Autodesk Inventor part; units mm, degrees
ref_plane "YZ Plane" through (0, 0, 0) normal (1, 0, 0) x (0, 1, 0)
ref_plane "XZ Plane" through (0, 0, 0) normal (0, 1, 0) x (-1, 0, 0)
ref_plane "XY Plane" through (0, 0, 0) normal (0, 0, 1) x (1, 0, 0)
sketch "Sketch4" plane through (0, 0, 0) normal (0, 0, 1) x (1, 0, 0)
  line L0 (0, 0) -> (1.5, 0)
  line L1 (1.5, 0) -> (1.5, -1)
  line L2 (1.5, -1) -> (2.5, -1)
  line L3 (2.5, -1) -> (2.5, 1)
  line L4 (2.5, 1) -> (0, 1)
  line L5 (0, 1) -> (0, 0)
  dimension "d22" = 1.5
  dimension "d23" = 1
  dimension "d24" = 1
  dimension "d25" = 2
extrude "Extrusion4" add sketch "Sketch4" along normal blind 10
sketch "Sketch5" plane through (1.5, -1, 0) normal (0, -1, 0) x (1, 0, 0)
  line L0 (0, 0) -> (1, 0)
  line L1 (1, 0) -> (1, 10)
  line L2 (0, 10) -> (1, 10)
  line L3 (0, 0) -> (0, 10)
  point P0 (-1.5, 0)
extrude "Extrusion5" add sketch "Sketch5" along normal blind 3.5
sketch "Sketch6" plane through (0, 0, 0) normal (-1, 0, 0) x (0, 0, 1)
  line L0 (0, 0) -> (10, 0)
  line L1 (1.29, 0.8) -> (1.69, 0.8)
  line L2 (1.69, 0.8) -> (1.69, 0.2)
  line L3 (1.69, 0.2) -> (1.29, 0.2)
  line L4 (1.29, 0.2) -> (1.29, 0.8)
  line L5 (3.63, 0.8) -> (4.03, 0.8)
  line L6 (4.03, 0.8) -> (4.03, 0.2)
  line L7 (4.03, 0.2) -> (3.63, 0.2)
  line L8 (3.63, 0.2) -> (3.63, 0.8)
  line L9 (5.97, 0.8) -> (6.37, 0.8)
  line L10 (6.37, 0.8) -> (6.37, 0.2)
  line L11 (6.37, 0.2) -> (5.97, 0.2)
  line L12 (5.97, 0.2) -> (5.97, 0.8)
  line L13 (0, 1) -> (0, 0)
  line L14 (10, 1) -> (10, 0)
  line L15 (8.31, 0.8) -> (8.71, 0.8)
  line L16 (8.71, 0.8) -> (8.71, 0.2)
  line L17 (8.71, 0.2) -> (8.31, 0.2)
  line L18 (8.31, 0.2) -> (8.31, 0.8)
  line L19 (0, 1) -> (10, 1)
  dimension "d30" = 0.4
  dimension "d31" = 0.6
  dimension "d32" = 0.4
  dimension "d33" = 0.6
  dimension "d36" = 0.4
  dimension "d37" = 0.6
  dimension "d38" = 1.94
  dimension "d40" = 0.2
  dimension "d41" = 0.2
  dimension "d42" = 0.2
  dimension "d49" = 1.29
  dimension "d50" = 1.94
  dimension "d51" = 0.4
  dimension "d52" = 0.6
  dimension "d53" = 0.2
  dimension "d54" = 1.94
  dimension "d55" = 1.29
  dimension "d80" = 0.2
extrude "Extrusion6" add sketch "Sketch6" along normal blind 3.5 contours L1 L2 L3 L4 | L5 L6 L7 L8 | L9 L10 L11 L12 | L15 L16 L17 L18
chamfer "Chamfer5" distance 0.15 distance2 0.5 1 edges at (-3.5, 0.2, 1.49) measured on face at (-3.5, 0.6, 1.4233)
chamfer "Chamfer6" distance 0.15 distance2 0.5 1 edges at (-3.5, 0.8, 1.49) measured on face at (-3.5, 0.65, 1.4233)
chamfer "Chamfer7" distance 0.15 distance2 0.5 1 edges at (-3.5, 0.2, 3.83) measured on face at (-3.5, 0.6, 3.7633)
chamfer "Chamfer8" distance 0.15 distance2 0.5 1 edges at (-3.5, 0.8, 3.83) measured on face at (-3.5, 0.65, 3.7633)
chamfer "Chamfer9" distance 0.15 distance2 0.5 1 edges at (-3.5, 0.2, 6.17) measured on face at (-3.5, 0.6, 6.1033)
chamfer "Chamfer10" distance 0.15 distance2 0.5 1 edges at (-3.5, 0.8, 6.17) measured on face at (-3.5, 0.65, 6.1033)
chamfer "Chamfer11" distance 0.15 distance2 0.5 1 edges at (-3.5, 0.8, 8.51) measured on face at (-3.5, 0.4, 8.5767)
chamfer "Chamfer12" distance 0.15 distance2 0.5 1 edges at (-3.5, 0.2, 8.51) measured on face at (-3.5, 0.35, 8.5767)
sketch "Sketch7" plane through (1.5, -4.5, 0) normal (0, -1, 0) x (1, 0, 0)
  line L0 (0, 10) -> (0, 0)
  line L1 (0.8, 8.71) -> (0.2, 8.71)
  line L2 (0.2, 8.71) -> (0.2, 8.31)
  line L3 (0.2, 8.31) -> (0.8, 8.31)
  line L4 (0.8, 8.31) -> (0.8, 8.71)
  line L5 (0.8, 6.37) -> (0.2, 6.37)
  line L6 (0.2, 6.37) -> (0.2, 5.97)
  line L7 (0.2, 5.97) -> (0.8, 5.97)
  line L8 (0.8, 5.97) -> (0.8, 6.37)
  line L9 (0.8, 4.03) -> (0.2, 4.03)
  line L10 (0.2, 4.03) -> (0.2, 3.63)
  line L11 (0.2, 3.63) -> (0.8, 3.63)
  line L12 (0.8, 3.63) -> (0.8, 4.03)
  line L13 (0.8, 1.69) -> (0.2, 1.69)
  line L14 (0.2, 1.69) -> (0.2, 1.29)
  line L15 (0.2, 1.29) -> (0.8, 1.29)
  line L16 (0.8, 1.29) -> (0.8, 1.69)
  point P0 (-1.5, 0)
  dimension "d81" = 0.6
  dimension "d82" = 0.4
  dimension "d83" = 0.4
  dimension "d84" = 0.4
  dimension "d85" = 0.4
  dimension "d86" = 0.2
extrude "Extrusion7" cut sketch "Sketch7" against normal blind 3.7
chamfer "Chamfer13" distance 0.15 angle 45 4 edges at (2, -4.5, 4.03) (2.3, -4.5, 3.83) (2, -4.5, 3.63) (1.7, -4.5, 3.83)
chamfer "Chamfer14" distance 0.15 angle 45 4 edges at (2, -4.5, 1.69) (2.3, -4.5, 1.49) (2, -4.5, 1.29) (1.7, -4.5, 1.49)
chamfer "Chamfer15" distance 0.15 angle 45 4 edges at (2.3, -4.5, 6.17) (2, -4.5, 6.37) (1.7, -4.5, 6.17) (2, -4.5, 5.97)
chamfer "Chamfer16" distance 0.15 angle 45 4 edges at (2, -4.5, 8.31) (2.3, -4.5, 8.51) (2, -4.5, 8.71) (1.7, -4.5, 8.51)
properties part number "Pin Connector Curved"
Verification items for the finished model (mm, model axes). A direction names the side the tool comes from. Coordinates: 2 decimals unless noted, no trailing zeros. Order: outer loops, then holes, each group sorted by start corner. A loop starts at its lowest first (then second) coordinate and runs counter-clockwise, first axis right, second up.
1. Sectioned sample at A-A, the plane y = -1. Record the cut outline in (x, z), and give its area (3 significant figures).
Results found:
outline: (1.5, 0) - (2.5, 0) - (2.5, 10) - (1.5, 10) - close; hole (1.7, 1.29) - (2.3, 1.29) - (2.3, 1.69) - (1.7, 1.69) - close; hole (1.7, 3.63) - (2.3, 3.63) - (2.3, 4.03) - (1.7, 4.03) - close; hole (1.7, 5.97) - (2.3, 5.97) - (2.3, 6.37) - (1.7, 6.37) - close; hole (1.7, 8.31) - (2.3, 8.31) - (2.3, 8.71) - (1.7, 8.71) - close
area: 9.04 mm2
2. Go/stop test with flat-tipped pins: pin 1 Ø1 at (x, z) = (-1, 7.5) entering from +Y; pin 2 Ø1.5 at (y, z) = (-3.5, 3.5) entering from -X; pin 3 Ø0.7 at (x, y) = (-2, 0.5) entering from +Z. Record where each tip stops, or that it passes through.
Results found:
pin 1: passes through
pin 2: stops at x = 1.5
pin 3: stops at z = 8.71
3. Sectioned sample at B-B, the plane x = -2.15. Record the cut outline in (y, z), and give its area (3 significant figures).
Results found:
outline: (0.2, 1.29) - (0.8, 1.29) - (0.8, 1.69) - (0.2, 1.69) - close; (0.2, 3.63) - (0.8, 3.63) - (0.8, 4.03) - (0.2, 4.03) - close; (0.2, 5.97) - (0.8, 5.97) - (0.8, 6.37) - (0.2, 6.37) - close; (0.2, 8.31) - (0.8, 8.31) - (0.8, 8.71) - (0.2, 8.71) - close
area: 0.960 mm2
4. Sectioned sample at D-D, the plane x = 0.3. Record the cut outline in (y, z).
Results found:
outline: (0, 0) - (1, 0) - (1, 10) - (0, 10) - close
5. Sectioned sample at C-C, the plane z = 5. Record the cut outline in (x, y), and give its area (3 significant figures).
Results found:
outline: (0, 0) - (1.5, 0) - (1.5, -4.5) - (2.5, -4.5) - (2.5, 1) - (0, 1) - close
area: 7.00 mm2
6. Release check for a two-part mould opening along Z. For faces 1 (the face through (2, -1, 0)), 2 (the face through (0, 0.5, 4.9)), 3 (the face through (2.5, -2, 5)), 4 (the face through (2, -1, 10)) record: +Z half, -Z half, draft (parallel to the pull), parting line (faces both ways), or undercut.
Results found:
face 1: -Z half
face 2: undercut
face 3: draft
face 4: +Z half
7. Scan lines: line 1 (Z direction, x = -1.95, y = 0.6); line 2 (X direction, y = -1.35, z = 1.5); line 3 (Y direction, x = 1.2, z = 8.75). Record each from-to range of solid material in increasing order.
Results found:
line 1: z = 1.29 to 1.69, 3.63 to 4.03, 5.97 to 6.37, 8.31 to 8.71
line 2: x = 1.5 to 1.7, 2.3 to 2.5
line 3: y = 0 to 1
8. Set-up check for faces 5 (the face through (1, 0, 5)), 6 (the face through (1, 1, 5)): record each of +Z, -Z, +X, -X, +Y, -Y from which the full face is reachable in a straight line by a thin tool's end or side.
Results found:
face 5: +Z, -Z, -X, -Y
face 6: +Z, -Z, +X, -X, +Y
